Could you check a few things on this drawing? It's one solid part, dimensions in mm from its lowest x, y, z. A direction names the side the tool comes from. Give positions to 0.01 mm unless a question says otherwise; leave off trailing zeros. Order: outer loops, then holes, each group sorted by start corner. A loop starts at its lowest first (then second) coordinate and runs counter-clockwise, first axis right, second up.
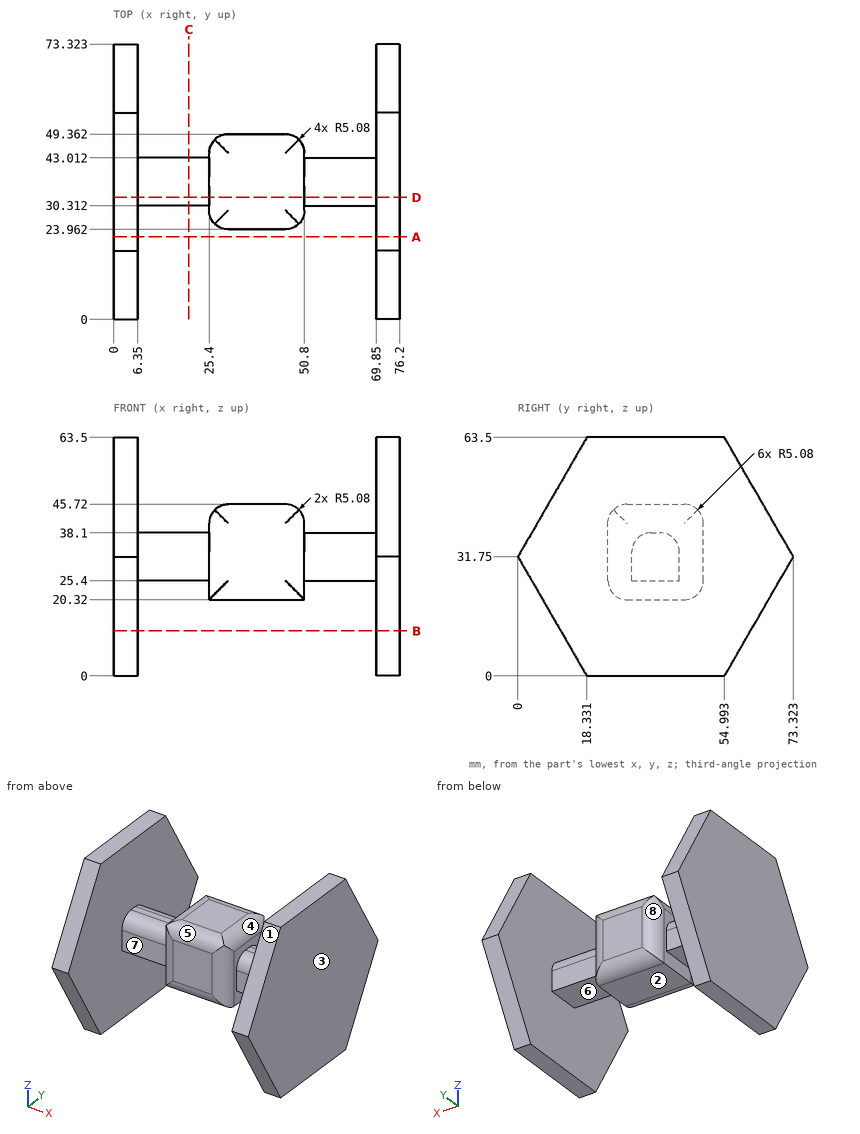
Q1. For the marked faces 4, 5, 6, 7 and 8, which set-ups out of +Z, -Z, +X, -X, +Y, -Y let a thin tool reach every point of the face, with its end or its side?
Filled sheet:
face 4: +Z, +Y, -Y
face 5: +Z, -Y
face 6: -Z, +Y, -Y
face 7: +Z, -Z, -Y
face 8: +Z, -Z, +Y
Q2. I'm going to push flat-ended pins straight in: P1, Ø8.5, axis at x = 12.5, z = 30, coming from the +Y side; P2, Ø0.8, axis at x = 64.5, y = 37, coming from the +Z side; P3, Ø4, axis at x = 63, y = 34, coming from the -Z side. Where does each tip first touch, or does it pass through?
Filled sheet:
P1: stops at y = 43.01
P2: stops at z = 38.1
P3: stops at z = 25.4
Q3. If we section it at D-D on y = 32.5: List the corners of the cut face in (x, z) for me.
Filled sheet:
outline: (0, 0) - (6.35, 0) - (6.35, 25.4) - (25.4, 25.4) - (25.4, 20.32) - (50.8, 20.32) - (50.8, 25.4) - (69.85, 25.4) - (69.85, 0) - (76.2, 0) - (76.2, 63.5) - (69.85, 63.5) - (69.85, 37.2) - (50.8, 37.2) - (50.8, 40.64) arc R5.08 ccw to (45.72, 45.72) - (30.48, 45.72) arc R5.08 ccw to (25.4, 40.64) - (25.4, 37.2) - (6.35, 37.2) - (6.35, 63.5) - (0, 63.5) - close
Q4. I need wall thicknesses on L1, parallel to X at y = 34.5, z = 39; L2, parallel to X at y = 69, z = 28; L3, parallel to Z at x = 32, y = 39. Which ranges of each line are inside material? Lowest first, please.
Filled sheet:
L1: x = 0 to 6.35, 25.4 to 50.8, 69.85 to 76.2
L2: x = 0 to 6.35, 69.85 to 76.2
L3: z = 20.32 to 45.72
Q5. If we section it at A-A on y = 22: List the corners of the cut face in (x, z) for me.
Filled sheet:
outline: (0, 0) - (6.35, 0) - (6.35, 63.5) - (0, 63.5) - close; (69.85, 0) - (76.2, 0) - (76.2, 63.5) - (69.85, 63.5) - close
Q6. Thinking about a two-plate mould opening in X: for the marked faces 1, 2 and 3, which applies, released by +X, released by -X, zero draft, split by the parting line, or undercut?
Filled sheet:
face 1: zero draft
face 2: undercut
face 3: released by +X
Q7. If we section it at B-B on z = 12: List the corners of the cut face in (x, y) for me.
Filled sheet:
outline: (0, 11.4) - (6.35, 11.4) - (6.35, 61.92) - (0, 61.92) - close; (69.85, 11.4) - (76.2, 11.4) - (76.2, 61.92) - (69.85, 61.92) - close
Q8. If we section it at C-C on x = 20: List the corners of the cut face in (y, z) for me.
Filled sheet:
outline: (30.31, 25.4) - (43.01, 25.4) - (43.01, 33.02) arc R5.08 ccw to (37.93, 38.1) - (35.39, 38.1) arc R5.08 ccw to (30.31, 33.02) - close
